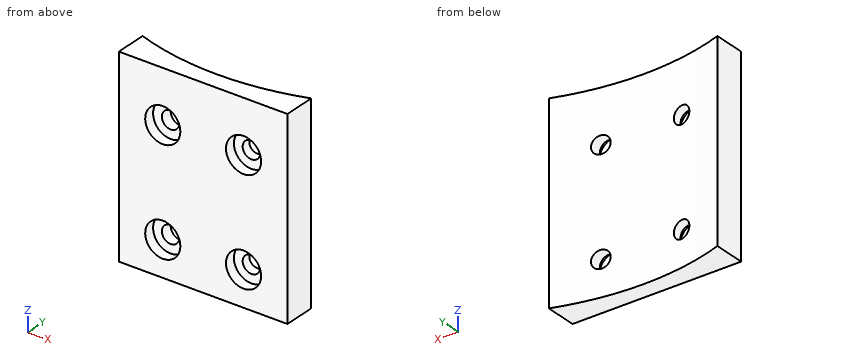
```python
from build123d import *

# Parameters (mm, degrees)
CYLINDER1836_R              = 5
CYLINDER1836_DEPTH          = 5
CYLINDER1839_R              = 5
CYLINDER1839_DEPTH          = 5
COMPOUND945_PLACEMENT_ANGLE = 90
CYLINDER1837_R              = 5
CYLINDER1837_DEPTH          = 5
CYLINDER1838_R              = 5
CYLINDER1838_DEPTH          = 5
COMPOUND944_PLACEMENT_ANGLE = 90
CYLINDER1834_R              = 2.5
CYLINDER1834_DEPTH          = 40
CYLINDER1835_R              = 2.5
CYLINDER1835_DEPTH          = 40
COMPOUND934_PLACEMENT_ANGLE = 90
CYLINDER1832_R              = 2.5
CYLINDER1832_DEPTH          = 40
CYLINDER1833_R              = 2.5
CYLINDER1833_DEPTH          = 40
COMPOUND933_PLACEMENT_ANGLE = 90
CYLINDER970_R               = 74
CYLINDER970_DEPTH           = 64
BOX481_W                    = 10
BOX481_H                    = 48
BOX481_DEPTH                = 55


with BuildPart() as obj1:
    # Cylinder1836 → Cylinder1836 (new body)
    with BuildSketch(Plane(origin=(-86, -10, 69), x_dir=(0, 0, -1), z_dir=(1, 0, 0))):
        Circle(CYLINDER1836_R)
    extrude(amount=CYLINDER1836_DEPTH)


with BuildPart() as compound945:
    # Cylinder1839 → Cylinder1839 (new body)
    with BuildSketch(Plane(origin=(-86, -10, 39), x_dir=(0, 0, -1), z_dir=(1, 0, 0))):
        Circle(CYLINDER1839_R)
    extrude(amount=CYLINDER1839_DEPTH)

    # Compound945: union obj1
    add(obj1.part)


with BuildPart() as compound945_1:
    # Compound945 placement: moved
    add(compound945.part.moved(Location((-21.5, 0, 0))).rotate(Axis((-21.5, 0, 0), (0, 0, 1)), COMPOUND945_PLACEMENT_ANGLE))


with BuildPart() as obj2:
    # Cylinder1837 → Cylinder1837 (new body)
    with BuildSketch(Plane(origin=(-86, -10, 69), x_dir=(0, 0, -1), z_dir=(1, 0, 0))):
        Circle(CYLINDER1837_R)
    extrude(amount=CYLINDER1837_DEPTH)


with BuildPart() as compound946:
    # Cylinder1838 → Cylinder1838 (new body)
    with BuildSketch(Plane(origin=(-86, -10, 39), x_dir=(0, 0, -1), z_dir=(1, 0, 0))):
        Circle(CYLINDER1838_R)
    extrude(amount=CYLINDER1838_DEPTH)

    # Compound944: union obj2
    add(obj2.part)


with BuildPart() as compound946_1:
    # Compound944 placement: moved
    add(compound946.part.moved(Location((1.5, 0, 0))).rotate(Axis((1.5, 0, 0), (0, 0, 1)), COMPOUND944_PLACEMENT_ANGLE))

    # Compound946: union Compound945
    add(compound945_1.part)


with BuildPart() as compound946_2:
    # Compound946 placement: moved
    add(compound946_1.part.moved(Location((0, 5, 0))))


with BuildPart() as obj3:
    # Cylinder1834 → Cylinder1834 (new body)
    with BuildSketch(Plane(origin=(-86, -10, 69), x_dir=(0, 0, -1), z_dir=(1, 0, 0))):
        Circle(CYLINDER1834_R)
    extrude(amount=CYLINDER1834_DEPTH)


with BuildPart() as compound934:
    # Cylinder1835 → Cylinder1835 (new body)
    with BuildSketch(Plane(origin=(-86, -10, 39), x_dir=(0, 0, -1), z_dir=(1, 0, 0))):
        Circle(CYLINDER1835_R)
    extrude(amount=CYLINDER1835_DEPTH)

    # Compound934: union obj3
    add(obj3.part)


with BuildPart() as compound934_1:
    # Compound934 placement: moved
    add(compound934.part.moved(Location((-21.5, 0, 0))).rotate(Axis((-21.5, 0, 0), (0, 0, 1)), COMPOUND934_PLACEMENT_ANGLE))


with BuildPart() as obj4:
    # Cylinder1832 → Cylinder1832 (new body)
    with BuildSketch(Plane(origin=(-86, -10, 69), x_dir=(0, 0, -1), z_dir=(1, 0, 0))):
        Circle(CYLINDER1832_R)
    extrude(amount=CYLINDER1832_DEPTH)


with BuildPart() as compound939:
    # Cylinder1833 → Cylinder1833 (new body)
    with BuildSketch(Plane(origin=(-86, -10, 39), x_dir=(0, 0, -1), z_dir=(1, 0, 0))):
        Circle(CYLINDER1833_R)
    extrude(amount=CYLINDER1833_DEPTH)

    # Compound933: union obj4
    add(obj4.part)


with BuildPart() as compound939_1:
    # Compound933 placement: moved
    add(compound939.part.moved(Location((1.5, 0, 0))).rotate(Axis((1.5, 0, 0), (0, 0, 1)), COMPOUND933_PLACEMENT_ANGLE))

    # Compound939: union Compound934
    add(compound934_1.part)


with BuildPart() as obj5:
    # Cylinder970 → Cylinder970 (new body)
    with BuildSketch(Plane.XY.offset(27)):
        Circle(CYLINDER970_R)
    extrude(amount=CYLINDER970_DEPTH)


with BuildPart() as cut596:
    # Box481 → Box481 (new body)
    with BuildSketch(Plane(origin=(24, -79, 29), x_dir=(0, 1, 0), z_dir=(0, 0, 1))):
        with Locations((5, 24)):
            Rectangle(BOX481_W, BOX481_H)
    extrude(amount=BOX481_DEPTH)

    # Cut450: cut obj5
    add(obj5.part, mode=Mode.SUBTRACT)

    # Cut595: cut Compound939
    add(compound939_1.part, mode=Mode.SUBTRACT)

    # Cut596: cut Compound946
    add(compound946_2.part, mode=Mode.SUBTRACT)


solid = cut596.part
```
Could you check a few things on this model? Use its own coordinates, in mm. Give positions to 0.01 mm unless a question says otherwise; leave off trailing zeros. Loops run counter-clockwise (first coordinate to the right, second up) from the corner with the lowest first, then second, coordinate; pieces in that order, holes last. Notation, with made-up numbers: (12.5, -21.5) - (16.5, -21.5) arc R18 cw to (16.5, -14.5) - close; hole circle Ø3 at (50, 41.5). An arc over 180 degrees is marked (long way). Use one line per item in the form item = value.
1. I want a section at D-D (z = 46.5). Please give me the cut outline in (x, y).
Response values:
outline = (-24, -79) - (24, -79) - (24, -70) arc R74 cw to (-24, -70) - close
2. I want a section at B-B (z = 69). Please give me the cut outline in (x, y), and give its area (3 significant figures).
Response values:
outline = (-24, -79) - (-16.5, -79) - (-16.5, -76) - (-14, -76) - (-14, -72.66) arc R74 cw to (-24, -70) - close; (-9, -76) - (-6.5, -76) - (-6.5, -79) - (6.5, -79) - (6.5, -76) - (9, -76) - (9, -73.45) arc R74 cw to (-9, -73.45) - close; (14, -76) - (16.5, -76) - (16.5, -79) - (24, -79) - (24, -70) arc R74 cw to (14, -72.66) - close
area = 214 mm²
3. I want a section at C-C (x = 0). Please give me the cut outline in (y, z).
Response values:
outline = (-79, 29) - (-74, 29) - (-74, 84) - (-79, 84) - close
4. I'm going to push flat-ended pins straight in: pin 1 Ø6 at (x, z) = (-11.5, 39) entering from +Y; pin 2 Ø8 at (x, z) = (-11.5, 69) entering from +Y; pin 3 Ø9 at (x, z) = (-11.5, 69) entering from +Y. Where does each tip first touch, or does it pass through?
Response values:
pin_1 = -72.57
pin_2 = -72.36
pin_3 = -72.25
5. I want a section at A-A (x = -11.5). Please give me the cut outline in (y, z), and give its area (3 significant figures).
Response values:
outline = (-79, 29) - (-73.1, 29) - (-73.1, 36.5) - (-76, 36.5) - (-76, 34) - (-79, 34) - close; (-79, 44) - (-76, 44) - (-76, 41.5) - (-73.1, 41.5) - (-73.1, 66.5) - (-76, 66.5) - (-76, 64) - (-79, 64) - close; (-79, 74) - (-76, 74) - (-76, 71.5) - (-73.1, 71.5) - (-73.1, 84) - (-79, 84) - close
area = 235 mm²
6. I need wall thicknesses on probe 1 along X at (y, z) = (-74.2, 69); probe 2 along Z at (x, y) = (11.5, -77.4); probe 3 along X at (y, z) = (-78.1, 69). Which ranges of each line are inside material? Lowest first, please.
Response values:
probe_1 = -24 to -14, -9 to 9, 14 to 24
probe_2 = 29 to 34, 44 to 64, 74 to 84
probe_3 = -24 to -16.5, -6.5 to 6.5, 16.5 to 24
